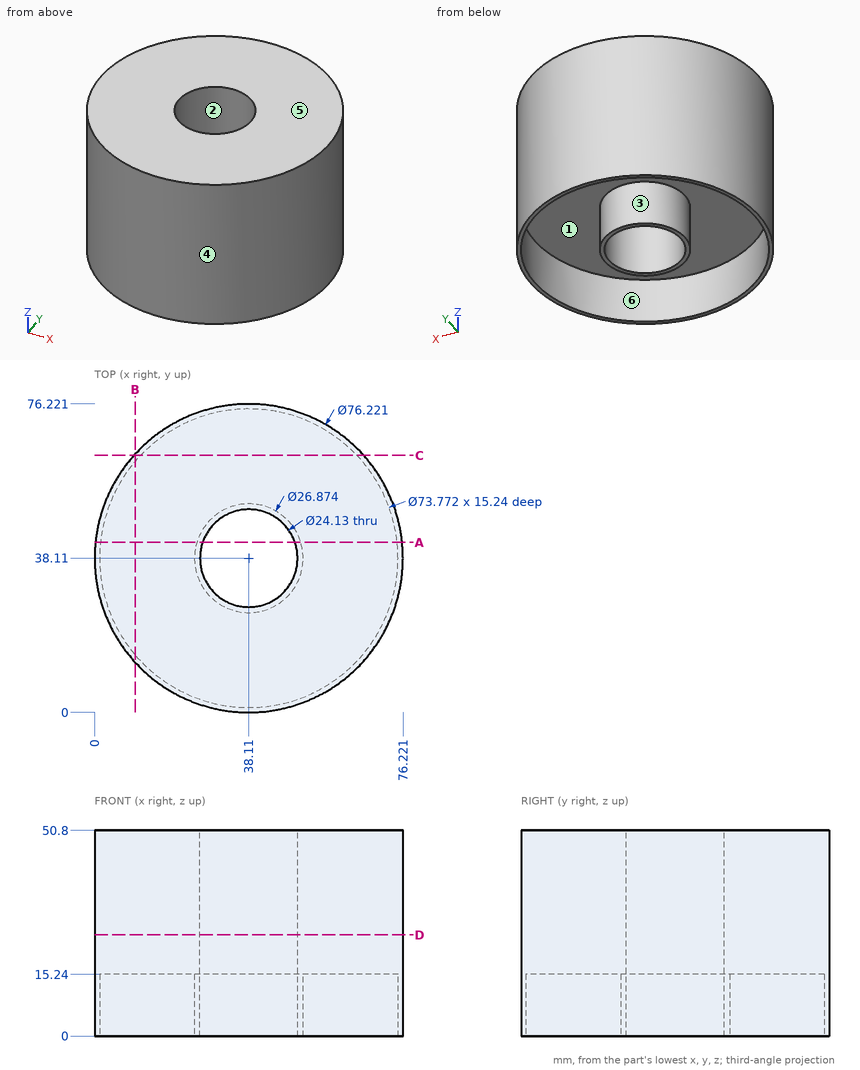
Study the drawing (mm; zero at the part's minimum x, y, z) and answer. A direction names the side the tool comes from. Round coordinates to 2 decimals unless told otherwise and drop trailing zeros. Loops run counter-clockwise (first coordinate to the right, second up) from the corner with the lowest first, then second, coordinate; pieces in that order, holes last. Notation, with made-up numbers: (-16.5, 32.25) - (2.5, 32.25) arc R9 cw to (2.5, 43.25) - close; hole circle Ø5 at (48.25, -9.5). An arc over 180 degrees is marked (long way). Use one line per item in the form item = value. Start each with the question number.
1. Given pin 1 Ø10 at (y, z) = (48.5, 24) entering from -X; pin 2 Ø2 at (x, y) = (51, 24) entering from -Z; pin 3 Ø3 at (y, z) = (12, 36) entering from -X; pin 4 Ø21.5 at (x, y) = (38.11, 38.11) entering from +Z, each flat-ended and moving along its own axis, determine where each tip first touches the part or whether it passes through.
2. For a pull along X with two mould halves and no side action, classify the marked faces 3, 4, 5 and 6 as pulls with the +X half, pulls with the -X half, needs draft (parallel to the pull), parting line crosses it, or undercut.
3. A tool of negligible diameter and unlimited length cuts with its end or side. For the marked faces 1 and 2, from which of +Z, -Z, +X, -X, +Y, -Y can it reach the whole face along a straight path? Write none if from no direction.
4. The part is cut by section A-A on y = 42. Determine the outline of the cut face in (x, z), then the cut area to 3 significant figures.
5. The part is cut by section B-B on x = 10. Determine the outline of the cut face in (y, z), then the cut area to 3 significant figures.
6. Consider line 1 (Y direction, x = 38, z = 14) (1 decimal); line 2 (X direction, y = 46.5, z = 3) (1 decimal); line 3 (Y direction, x = 7, z = 3) (1 decimal). Determine where each line is inside the solid, lowest interval first. Write a range as [from, to].
7. The part is cut by section D-D on z = 25. Determine the outline of the cut face in (x, y) (1 decimal), then the cut area to 3 significant figures.
8. The part is cut by section C-C on y = 63.5. Determine the outline of the cut face in (x, z), then the cut area to 3 significant figures.
Geometry check:
q1.pin_1 = 0.38
q1.pin_2 = 15.24
q1.pin_3 = 9.01
q1.pin_4 = through
q2.face_3 = undercut
q2.face_4 = parting line crosses it
q2.face_5 = needs draft
q2.face_6 = undercut
q3.face_1 = -Z
q3.face_2 = +Z, -Z
q4.outline = (0.2, 0) - (1.43, 0) - (1.43, 15.24) - (25.25, 15.24) - (25.25, 0) - (26.69, 0) - (26.69, 50.8) - (0.2, 50.8) - close; (49.53, 0) - (50.97, 0) - (50.97, 15.24) - (74.79, 15.24) - (74.79, 0) - (76.02, 0) - (76.02, 50.8) - (49.53, 50.8) - close
q4.area = 1,970 mm^2
q5.outline = (12.38, 0) - (14.23, 0) - (14.23, 15.24) - (61.99, 15.24) - (61.99, 0) - (63.84, 0) - (63.84, 50.8) - (12.38, 50.8) - close
q5.area = 1,890 mm^2
q6.line_1 = [0, 1.2], [24.7, 26], [50.2, 51.5], [75, 76.2]
q6.line_2 = [0.9, 2.2], [27.6, 29.4], [46.8, 48.6], [74, 75.3]
q6.line_3 = [16.1, 18.3], [57.9, 60.1]
q7.outline = circle Ø76.2 at (38.1, 38.1); hole circle Ø24.1 at (38.1, 38.1)
q7.area = 4,110 mm^2
q8.outline = (9.69, 0) - (11.35, 0) - (11.35, 15.24) - (64.87, 15.24) - (64.87, 0) - (66.53, 0) - (66.53, 50.8) - (9.69, 50.8) - close
q8.area = 2,070 mm^2
